from build123d import *

# Parameters (mm, degrees)
SKETCH2_R                            = 2.0193
BOSS_EXTRUDE1_DEPTH                  = 307.975
F_10_32_TAPPED_HOLE2_D               = 4.0386
F_10_32_TAPPED_HOLE2_DEPTH           = 16.34744
F_10_32_TAPPED_HOLE2_TIP             = 1.213317848
F_10_32_TAPPED_HOLE2_ON_FACE_2_D     = 4.0386
F_10_32_TAPPED_HOLE2_ON_FACE_2_DEPTH = 16.34744
F_10_32_TAPPED_HOLE2_ON_FACE_2_TIP   = 1.213317848


with BuildPart() as part:
    # Sketch2 → Boss-Extrude1 (new, symmetric)
    with BuildSketch(Plane.XY):
        with BuildLine():
            ThreePointArc((0.741687758, 5.071047688), (0, 5.125000037), (-0.741687758, 5.071047688))
            Line((-0.741687758, 5.071047688), (-4.020812242, 3.177844283))
            ThreePointArc((-4.020812242, 3.177844283), (-4.438380226, 2.562500019), (-4.7625, 1.893203404))
            Line((-4.7625, 1.893203404), (-4.7625, -1.893203404))
            ThreePointArc((-4.7625, -1.893203404), (-4.438380226, -2.562500019), (-4.020812242, -3.177844283))
            Line((-4.020812242, -3.177844283), (-0.741687758, -5.071047688))
            ThreePointArc((-0.741687758, -5.071047688), (0, -5.125000037), (0.741687758, -5.071047688))
            Line((0.741687758, -5.071047688), (4.020812242, -3.177844283))
            ThreePointArc((4.020812242, -3.177844283), (4.438380226, -2.562500019), (4.7625, -1.893203404))
            Line((4.7625, -1.893203404), (4.7625, 1.893203404))
            ThreePointArc((4.7625, 1.893203404), (4.438380226, 2.562500019), (4.020812242, 3.177844283))
            Line((4.020812242, 3.177844283), (0.741687758, 5.071047688))
        make_face()
        Circle(SKETCH2_R, mode=Mode.SUBTRACT)
    extrude(amount=BOSS_EXTRUDE1_DEPTH, both=True)

    # #10-32 Tapped Hole2
    with Locations(Plane(origin=(0, 0, -307.975), x_dir=(-1, 0, 0), z_dir=(0, 0, -1))):
        with Locations((0, 0)):
            Hole(F_10_32_TAPPED_HOLE2_D / 2, depth=F_10_32_TAPPED_HOLE2_DEPTH)
            with Locations((0, 0, -(F_10_32_TAPPED_HOLE2_DEPTH + F_10_32_TAPPED_HOLE2_TIP / 2))):  # 118° drill point
                Cone(0, F_10_32_TAPPED_HOLE2_D / 2, F_10_32_TAPPED_HOLE2_TIP, mode=Mode.SUBTRACT)

    # #10-32 Tapped Hole2 on face 2
    with Locations(Plane(origin=(0, 0, 307.975), x_dir=(-1, 0, 0), z_dir=(0, 0, -1))):
        with Locations((0, 0)):
            Hole(F_10_32_TAPPED_HOLE2_ON_FACE_2_D / 2, depth=F_10_32_TAPPED_HOLE2_ON_FACE_2_DEPTH)
            with Locations((0, 0, -(F_10_32_TAPPED_HOLE2_ON_FACE_2_DEPTH + F_10_32_TAPPED_HOLE2_ON_FACE_2_TIP / 2))):  # 118° drill point
                Cone(0, F_10_32_TAPPED_HOLE2_ON_FACE_2_D / 2, F_10_32_TAPPED_HOLE2_ON_FACE_2_TIP, mode=Mode.SUBTRACT)


solid = part.part
Could you check a few things on this model? Use its own coordinates, in mm. Give positions to 0.01 mm unless a question says otherwise; leave off trailing zeros. Order: outer loops, then holes, each group sorted by start corner. A loop starts at its lowest first (then second) coordinate and runs counter-clockwise, first axis right, second up.
1. Suppose I cut it at A-A (y = 0). List the corners of the cut face in (x, z) for me (1 decimal), plus the area to 3 significant figures.
2. I need wall thicknesses on L1, parallel to X at y = 1.75, z = -126.5; L2, parallel to Y at x = -1.5, z = 256; L3, parallel to X at y = 1.25, z = -207. Which ranges of each line are inside material? Lowest first, please.
3. Will these pins go through, and if not, where does the flat tip stop? P1, Ø1.5, axis at y = -3, z = 166.5, coming from the +X side; P2, Ø1, axis at x = 1, z = 70.5, coming from the +Y side.
Solved:
1. outline: (-4.8, -308) - (-2, -308) - (-2, 308) - (-4.8, 308) - close; (2, -308) - (4.8, -308) - (4.8, 308) - (2, 308) - close
1. area: 3,380 mm2
2. L1: x = -4.76 to -1.01, 1.01 to 4.76
2. L2: y = -4.63 to -1.35, 1.35 to 4.63
2. L3: x = -4.76 to -1.59, 1.59 to 4.76
3. P1: stops at x = 4.6
3. P2: stops at y = 5.1
